Check sheet for the drawn part. Datum: minimum x, y, z corner. Units: mm. A direction names the side the tool comes from. Round coordinates to 2 decimals unless told otherwise and drop trailing zeros. Order: outer loops, then holes, each group sorted by start corner. A loop starts at its lowest first (then second) coordinate and runs counter-clockwise, first axis right, second up. Notation, with made-up numbers: (42, 28) -> (98, 28) arc R8 cw to (98, 40) -> close; hole circle Ø6 at (15.5, 59). An arc over 180 degrees is marked (long way). Answer in a Markdown table with one row per item.
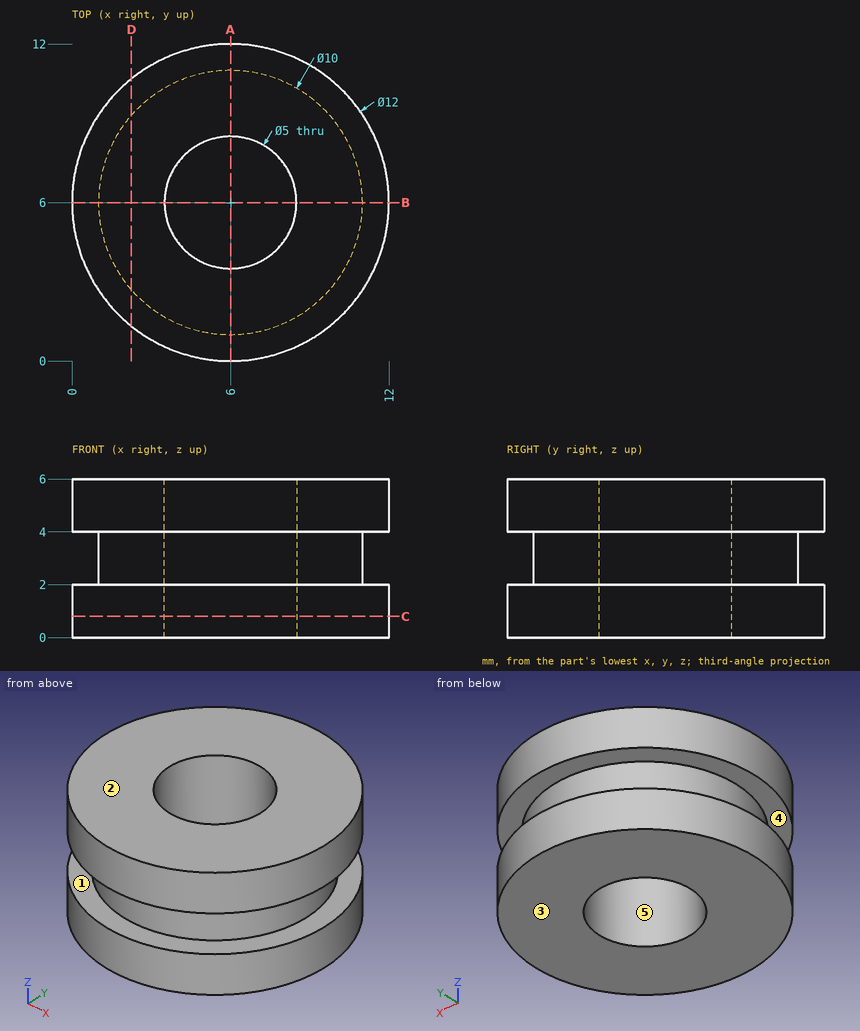
(1) Section check C-C on z = 0.8. Record the boundary of the cut face in (x, y), plus the area to 3 significant figures.
Solutions:
| item | result |
|---|---|
| outline | circle Ø12 at (6, 6); hole circle Ø5 at (6, 6) |
| area | 93.5 mm^2 |
(2) Draft check along Z on the marked faces 3, 4 and 5. Enter one of: pulls with the +Z half, pulls with the -Z half, needs draft (parallel to the pull), parting line crosses it, or undercut.
Solutions:
| item | result |
|---|---|
| face 3 | pulls with the -Z half |
| face 4 | undercut |
| face 5 | needs draft |
(3) Scan lines: probe 1 along Y at (x, z) = (6, 2.75); probe 2 along Z at (x, y) = (6.75, 11.25); probe 3 along Y at (x, z) = (5.25, 0.3). Record each from-to range of solid material in increasing order. Write a range as from..to.
Solutions:
| item | result |
|---|---|
| probe 1 | 1..3.5, 8.5..11 |
| probe 2 | 0..2, 4..6 |
| probe 3 | 0.05..3.62, 8.38..11.95 |
(4) Section check A-A on x = 6. Record the boundary of the cut face in (y, z).
Solutions:
| item | result |
|---|---|
| outline | (0, 0) -> (3.5, 0) -> (3.5, 6) -> (0, 6) -> (0, 4) -> (1, 4) -> (1, 2) -> (0, 2) -> close; (8.5, 0) -> (12, 0) -> (12, 2) -> (11, 2) -> (11, 4) -> (12, 4) -> (12, 6) -> (8.5, 6) -> close |
(5) Tool access check on the marked faces 1 and 2. Record the directions out of +Z, -Z, +X, -X, +Y, -Y that give a thin tool (end or side, any length) a straight path to the whole face; none if there is none.
Solutions:
| item | result |
|---|---|
| face 1 | none |
| face 2 | +Z, +X, -X, +Y, -Y |
(6) Depth check by flat-ended pin: pin 1 Ø1.5 at (y, z) = (8.5, 1) entering from -X. Enter the tip coordinate at first touch or a pass-through.
Solutions:
| item | result |
|---|---|
| pin 1 | x = 0.26 |
(7) Section check D-D on x = 2.25. Record the boundary of the cut face in (y, z), plus the area to 3 significant figures.
Solutions:
| item | result |
|---|---|
| outline | (1.32, 0) -> (10.68, 0) -> (10.68, 2) -> (9.31, 2) -> (9.31, 4) -> (10.68, 4) -> (10.68, 6) -> (1.32, 6) -> (1.32, 4) -> (2.69, 4) -> (2.69, 2) -> (1.32, 2) -> close |
| area | 50.7 mm^2 |
